from build123d import *

# Parameters (mm, degrees)
SKETCH1_R           = 20
SKETCH1_R_2         = 1.15
BOSS_EXTRUDE1_DEPTH = 3.18


with BuildPart() as part:
    # Sketch1 → Boss-Extrude1 (new body)
    with BuildSketch(Plane.XY):
        Circle(SKETCH1_R)
        Circle(SKETCH1_R_2, mode=Mode.SUBTRACT)
        with Locations((-8, 0)):
            Circle(SKETCH1_R_2, mode=Mode.SUBTRACT)
        with Locations((8, 0)):
            Circle(SKETCH1_R_2, mode=Mode.SUBTRACT)
        with BuildLine():
            Line((-1.5, 18.188251703), (-1.5, 3.621320344))
            Line((-1.5, 3.621320344), (-11.800375945, 13.921696289))
            ThreePointArc((-11.800375945, 13.921696289), (-6.983972641, 16.860801468), (-1.5, 18.188251703))
        make_face(mode=Mode.SUBTRACT)
        with BuildLine():
            Line((-1.5, -3.621320344), (-1.5, -18.188251703))
            ThreePointArc((-1.5, -18.188251703), (-6.983972641, -16.860801468), (-11.800375945, -13.921696289))
            Line((-11.800375945, -13.921696289), (-1.5, -3.621320344))
        make_face(mode=Mode.SUBTRACT)
        with BuildLine():
            Line((1.5, -3.621320344), (1.5, -18.188251703))
            ThreePointArc((1.5, -18.188251703), (6.983972641, -16.860801468), (11.800375945, -13.921696289))
            Line((11.800375945, -13.921696289), (1.5, -3.621320344))
        make_face(mode=Mode.SUBTRACT)
        with BuildLine():
            Line((1.5, 18.188251703), (1.5, 3.621320344))
            Line((1.5, 3.621320344), (11.800375945, 13.921696289))
            ThreePointArc((11.800375945, 13.921696289), (6.983972641, 16.860801468), (1.5, 18.188251703))
        make_face(mode=Mode.SUBTRACT)
        with BuildLine():
            Line((-18.188251703, 1.5), (-3.621320344, 1.5))
            Line((-3.621320344, 1.5), (-13.921696289, 11.800375945))
            ThreePointArc((-13.921696289, 11.800375945), (-16.860801468, 6.983972641), (-18.188251703, 1.5))
        make_face(mode=Mode.SUBTRACT)
        with BuildLine():
            Line((-18.188251703, -1.5), (-3.621320344, -1.5))
            Line((-3.621320344, -1.5), (-13.921696289, -11.800375945))
            ThreePointArc((-13.921696289, -11.800375945), (-16.860801468, -6.983972641), (-18.188251703, -1.5))
        make_face(mode=Mode.SUBTRACT)
        with BuildLine():
            Line((3.621320344, 1.5), (18.188251703, 1.5))
            ThreePointArc((18.188251703, 1.5), (16.860801468, 6.983972641), (13.921696289, 11.800375945))
            Line((13.921696289, 11.800375945), (3.621320344, 1.5))
        make_face(mode=Mode.SUBTRACT)
        with BuildLine():
            Line((3.621320344, -1.5), (18.188251703, -1.5))
            ThreePointArc((18.188251703, -1.5), (16.860801468, -6.983972641), (13.921696289, -11.800375945))
            Line((13.921696289, -11.800375945), (3.621320344, -1.5))
        make_face(mode=Mode.SUBTRACT)
    extrude(amount=BOSS_EXTRUDE1_DEPTH)


solid = part.part
Can you work these out from the model? Positions are in its coordinate system, mm. A direction names the side the tool comes from. Give positions to 0.01 mm unless a question says otherwise; leave off trailing zeros. Write each loop counter-clockwise with the first axis right and the second up, starting at its lowest first coordinate (ties: lowest second). Pieces come first, ordered by that corner, then holes. Notation, with made-up numbers: (31, -16) -> (35, -16) arc R21 ccw to (35, 0) -> close; hole circle Ø2 at (65, 70.5). An arc over 180 degrees is marked (long way). Answer as a JSON object with one key per item and string values. Group by question number.
Item 1: Suppose I cut it at B-B (x = 0). Please give me the cut outline in (y, z), plus the area to 3 significant figures.
Item 2: Suppose I cut it at D-D (y = 16.5). Please give me the cut outline in (x, z), plus the area to 3 significant figures.
Item 3: Please list where these lines run through material, in increasing order: line 1 (Y direction, x = 8, z = 2.1); line 2 (X direction, y = 14, z = 1.8); line 3 (X direction, y = 7.5, z = 0.6). Write a range as [from, to].
Item 4: For faces 4 (the face through (-5, 0, 0)), 5 (the face through (-8.7, 6.58, 1.57)), which set-ups out of +Z, -Z, +X, -X, +Y, -Y let a thin tool reach every point of the face, with its end or its side?
Item 5: We'd pull the mould along Y, two halves only. Please class faces 1 (the face through (-5, 0, 3.18)), 2 (the face through (-4.336, -19.524, 1.568)), 3 (the face through (6.91, -16.89, 1.57)): +Y half, -Y half, draft (parallel to the pull), parting line (faces both ways), or undercut.
Item 6: Suppose I cut it at C-C (z = 0.65). State how many separate pieces and enclosed holes the cut face has, plus the area to 3 significant figures.
Item 7: I'm going to push flat-ended pins straight in: P1, Ø5, axis at x = -13, y = 15.5, coming from the -Z side; P2, Ø1, axis at x = 13.5, z = 1.5, coming from the -Y side; P3, Ø1.6, axis at x = 13.5, z = 2, coming from the +Y side; P4, Ø1, axis at y = 10.5, z = 1.5, coming from the +X side. Where does each tip first touch, or does it pass through?
Item 8: Suppose I cut it at A-A (y = 0). Please give me the cut outline in (x, z), plus the area to 3 significant figures.
Findings:
{
 "1": {"outline": "(-20, 0) -> (-1.15, 0) -> (-1.15, 3.18) -> (-20, 3.18) -> close; (1.15, 0) -> (20, 0) -> (20, 3.18) -> (1.15, 3.18) -> close", "area": "120 mm²"},
 "2": {"outline": "(-11.3, 0) -> (-7.8, 0) -> (-7.8, 3.18) -> (-11.3, 3.18) -> close; (-1.5, 0) -> (1.5, 0) -> (1.5, 3.18) -> (-1.5, 3.18) -> close; (7.8, 0) -> (11.3, 0) -> (11.3, 3.18) -> (7.8, 3.18) -> close", "area": "31.8 mm²"},
 "3": {"line 1": "y = [-18.33, -16.4], [-10.12, -5.88], [-1.5, -1.15], [1.15, 1.5], [5.88, 10.12], [16.4, 18.33]", "line 2": "x = [-14.28, -11.71], [-1.5, 1.5], [11.71, 14.28]", "line 3": "x = [-18.54, -16.64], [-9.62, -5.38], [-1.5, 1.5], [5.38, 9.62], [16.64, 18.54]"},
 "4": {"face 4": "-Z, +X, -X, +Y, -Y", "face 5": "+Z, -Z"},
 "5": {"face 1": "draft", "face 2": "parting line", "face 3": "undercut"},
 "6": {"separate pieces": "1", "enclosed holes": "11", "area": "592 mm²"},
 "7": {"P1": "stops at z = 0", "P2": "stops at y = -15.2", "P3": "stops at y = 15.45", "P4": "stops at x = 17.32"},
 "8": {"outline": "(-20, 0) -> (-9.15, 0) -> (-9.15, 3.18) -> (-20, 3.18) -> close; (-6.85, 0) -> (-1.15, 0) -> (-1.15, 3.18) -> (-6.85, 3.18) -> close; (1.15, 0) -> (6.85, 0) -> (6.85, 3.18) -> (1.15, 3.18) -> close; (9.15, 0) -> (20, 0) -> (20, 3.18) -> (9.15, 3.18) -> close", "area": "105 mm²"}
}
